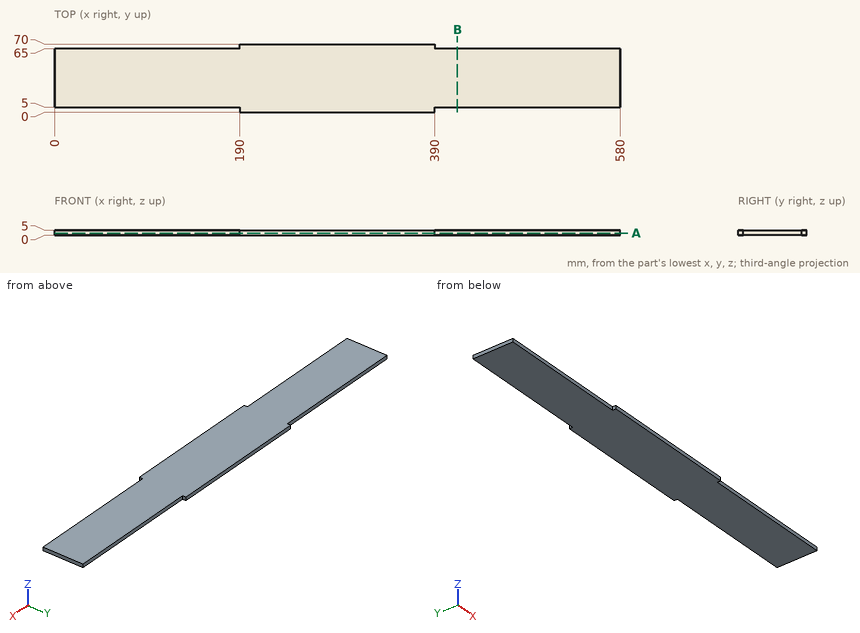
Answer from the drawing. Dimensions are ordinates in mm from the lowest x, y and z of the part. Round coordinates to 2 decimals unless told otherwise and drop trailing zeros. Write each loop counter-clockwise with the first axis right and the second up, starting at its lowest first coordinate (ties: lowest second). Pieces come first, ordered by that corner, then holes. Notation, with made-up numbers: M 11.25,21 L 57.25,21 A11 cw 57.25,40 Z; hole C 12,40.25 d1. An arc over 180 degrees is marked long. Write each question's results on one line, items separated by ' | '. Start each with the question number.
Item 1: Find section A-A on z = 2.1. Write down the section's boundary in (x, y).
Item 2: Given pin 1 Ø1.5 at (x, z) = (55, 3.5) entering from -Y; pin 2 Ø1 at (x, y) = (279, 9) entering from -Z; pin 3 Ø1.5 at (y, z) = (2, 2.5) entering from -X; pin 4 Ø2.5 at (y, z) = (1.5, 2) entering from +X, each flat-ended and moving along its own axis, determine where each tip first touches the part or whether it passes through.
Item 3: A straight line is drawn through the part: probe 1 along Y at (x, z) = (530, 1). Find the intervals that lie inside material, in ascending order.
Item 4: Find section B-B on x = 413. Write down the section's boundary in (y, z), and give its area (3 significant figures).
Answer block:
1) outline: M 0,5 L 190,5 L 190,0 L 390,0 L 390,5 L 580,5 L 580,65 L 390,65 L 390,70 L 190,70 L 190,65 L 0,65 Z
2) pin 1: stops at y = 5 | pin 2: stops at z = 0 | pin 3: stops at x = 190 | pin 4: stops at x = 390
3) probe 1: y = 5 to 65
4) outline: M 5,0 L 65,0 L 65,5 L 5,5 Z | area: 300 mm²
